Input: dimensioned drawing with shaded views. Units: mm. Origin: part minimum x, y, z. A direction names the side the tool comes from. Give positions to 0.01 mm unless a question says otherwise; leave off trailing zeros. Write each loop counter-clockwise with the first axis right and the second up, starting at its lowest first coordinate (ties: lowest second). Pieces come first, ordered by that corner, then holes.
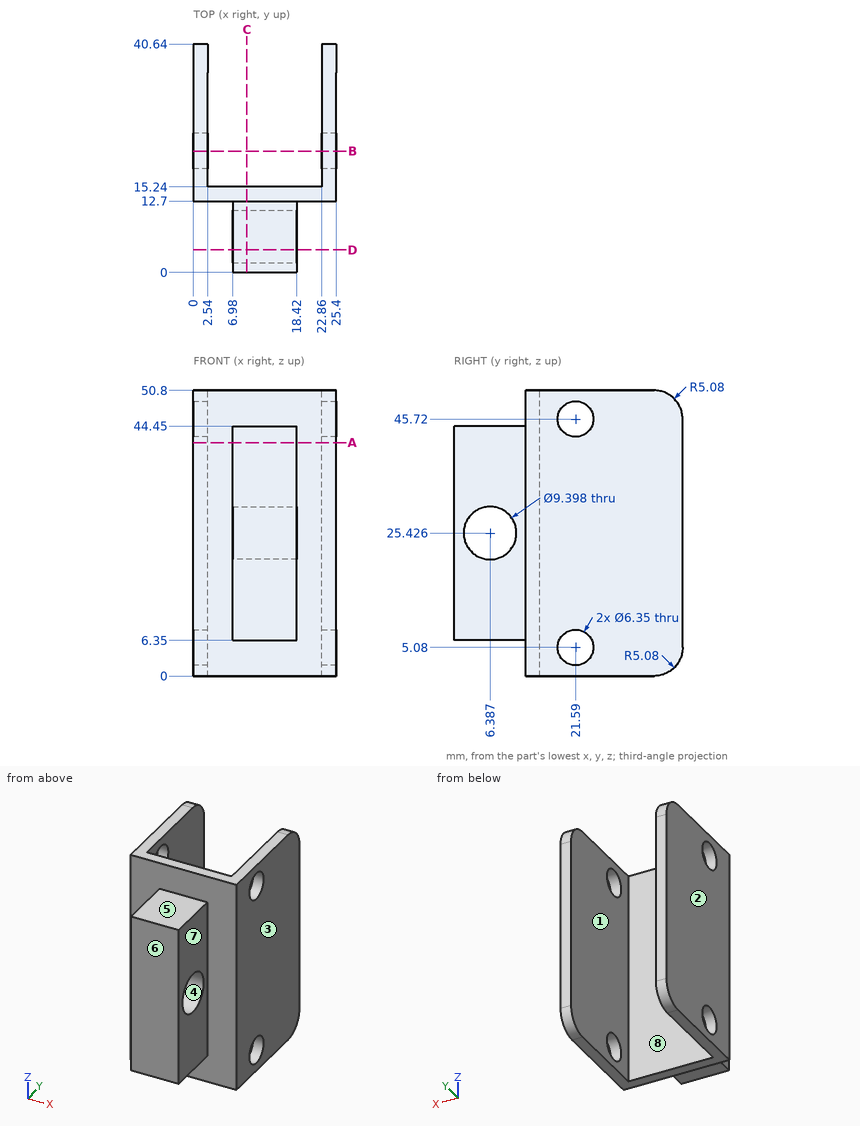
Item 1: Section D-D, the plane y = 4. Return the cut outline in (x, z), plus the area to 3 significant figures.
Found:
outline: (6.98, 6.35) - (18.42, 6.35) - (18.42, 21.38) - (6.98, 21.38) - close; (6.98, 29.47) - (18.42, 29.47) - (18.42, 44.45) - (6.98, 44.45) - close
area: 343 mm2
Item 2: Section C-C, the plane x = 9.5. Return the cut outline in (y, z).
Found:
outline: (0, 6.35) - (12.7, 6.35) - (12.7, 0) - (15.24, 0) - (15.24, 50.8) - (12.7, 50.8) - (12.7, 44.45) - (0, 44.45) - close; hole circle Ø9.4 at (6.39, 25.43)
Item 3: Line query: L1, parallel to X at y = 20, z = 31; L2, parallel to X at y = 5, z = 30.5; L3, parallel to Y at x = 10.25, z = 19. Output: solid intervals per line, ascending.
Found:
L1: x = 0 to 2.54, 22.86 to 25.4
L2: x = 6.98 to 18.42
L3: y = 0 to 15.24
Item 4: Pin query (flat end, axial travel): pin 1 Ø10 at (x, z) = (9.5, 25) entering from +Y; pin 2 Ø1.5 at (x, y) = (7.5, 7.5) entering from +Z; pin 3 Ø6.5 at (y, z) = (6, 21.5) entering from -X. Return the tip coordinate at first contact, or that it passes through.
Found:
pin 1: stops at y = 15.24
pin 2: stops at z = 44.45
pin 3: stops at x = 6.98
Item 5: Section A-A, the plane z = 41.5. Return the cut outline in (x, y), plus the area to 3 significant figures.
Found:
outline: (0, 12.7) - (6.98, 12.7) - (6.98, 0) - (18.42, 0) - (18.42, 12.7) - (25.4, 12.7) - (25.4, 40.64) - (22.86, 40.64) - (22.86, 15.24) - (2.54, 15.24) - (2.54, 40.64) - (0, 40.64) - close
area: 339 mm2
Item 6: Reachability of the marked faces 4, 5, 6, 7 and 8 from +Z, -Z, +X, -X, +Y, -Y: full face, straight path, thin tool, end or side. Return the list, or none.
Found:
face 4: +X, -X
face 5: +Z, +X, -X, -Y
face 6: +Z, -Z, +X, -X, -Y
face 7: +Z, -Z, +X, -Y
face 8: +Z, -Z, +Y
Item 7: Pull-direction query (X, two-part tool) for the marked faces 1, 2 and 3; classes: +X half, -X half, draft (parallel to the pull), parting line (faces both ways), or undercut.
Found:
face 1: undercut
face 2: -X half
face 3: +X half
Item 8: Section B-B, the plane y = 21.59. Return the cut outline in (x, z) (1 decimal).
Found:
outline: (0, 0) - (2.5, 0) - (2.5, 1.9) - (0, 1.9) - close; (0, 8.3) - (2.5, 8.3) - (2.5, 42.5) - (0, 42.5) - close; (0, 48.9) - (2.5, 48.9) - (2.5, 50.8) - (0, 50.8) - close; (22.9, 0) - (25.4, 0) - (25.4, 1.9) - (22.9, 1.9) - close; (22.9, 8.3) - (25.4, 8.3) - (25.4, 42.5) - (22.9, 42.5) - close; (22.9, 48.9) - (25.4, 48.9) - (25.4, 50.8) - (22.9, 50.8) - close
